from build123d import *

# Parameters (mm, degrees)
SKETCH_1_R      = 1.55
EXTRUDE_1_DEPTH = 2.1


with BuildPart() as part:
    # 草图1 → 凸台-拉伸1 (new body)
    with BuildSketch(Plane.XY):
        with BuildLine():
            Line((-13, -7.4), (13, -7.4))
            Line((13, -7.4), (13, 7.4))
            Line((13, 7.4), (7.1, 7.4))
            ThreePointArc((7.1, 7.4), (6.05, 6.35), (5, 7.4))
            Line((5, 7.4), (5, 9.5))
            Line((5, 9.5), (-5, 9.5))
            Line((-5, 9.5), (-5, 7.4))
            ThreePointArc((-5, 7.4), (-6.05, 6.35), (-7.1, 7.4))
            Line((-7.1, 7.4), (-13, 7.4))
            Line((-13, 7.4), (-13, -7.4))
        make_face()
        with BuildLine():
            ThreePointArc((-6.8, -3.05), (-7.10753788, -3.79246212), (-7.85, -4.1))
            Line((-7.85, -4.1), (-10.15, -4.1))
            ThreePointArc((-10.15, -4.1), (-11.2, -3.05), (-10.15, -2))
            Line((-10.15, -2), (-10.15, 1.8))
            ThreePointArc((-10.15, 1.8), (-11.2, 2.85), (-10.15, 3.9))
            Line((-10.15, 3.9), (-7.85, 3.9))
            ThreePointArc((-7.85, 3.9), (-7.10753788, 3.59246212), (-6.8, 2.85))
            ThreePointArc((-6.8, 2.85), (-7.10753788, 2.10753788), (-7.85, 1.8))
            Line((-7.85, 1.8), (-7.85, -2))
            ThreePointArc((-7.85, -2), (-7.10753788, -2.30753788), (-6.8, -3.05))
        make_face(mode=Mode.SUBTRACT)
        with Locations((0, 0.1)):
            Circle(SKETCH_1_R, mode=Mode.SUBTRACT)
        with BuildLine():
            ThreePointArc((7.85, 1.8), (6.8, 2.85), (7.85, 3.9))
            Line((7.85, 3.9), (10.15, 3.9))
            ThreePointArc((10.15, 3.9), (10.89246212, 3.59246212), (11.2, 2.85))
            ThreePointArc((11.2, 2.85), (10.89246212, 2.10753788), (10.15, 1.8))
            Line((10.15, 1.8), (10.15, -2))
            ThreePointArc((10.15, -2), (10.89246212, -2.30753788), (11.2, -3.05))
            ThreePointArc((11.2, -3.05), (10.89246212, -3.79246212), (10.15, -4.1))
            Line((10.15, -4.1), (7.85, -4.1))
            ThreePointArc((7.85, -4.1), (6.8, -3.05), (7.85, -2))
            Line((7.85, -2), (7.85, 1.8))
        make_face(mode=Mode.SUBTRACT)
    extrude(amount=EXTRUDE_1_DEPTH)


solid = part.part
Here's how the part is built. I have some questions about the finished solid (model axes, mm). A direction names the side the tool comes from. Coordinates: 2 decimals unless noted, no trailing zeros. Loops run counter-clockwise (first coordinate to the right, second up) from the corner with the lowest first, then second, coordinate; pieces in that order, holes last.
1. For P1, Ø0.6, axis at x = 9, z = 1, coming from the +Y side; P2, Ø0.6, axis at y = 8.5, z = 1, coming from the -X side, each with a flat end and sliding along its axis, tell me the tip position at first contact or that it passes through.
2. Imagine slicing it at A-A, the plane x = 0. Please give me the cut outline in (y, z), and give its area (3 significant figures).
3. Imagine slicing it at C-C, the plane y = 0.1. Please give me the cut outline in (x, z).
4. Imagine slicing it at D-D, the plane x = -6.05. Please give me the cut outline in (y, z).
5. I need wall thicknesses on L1, parallel to Y at x = -9.5, z = 1; L2, parallel to X at y = 1, z = 0.6; L3, parallel to Y at x = 0, z = 0.5. Which ranges of each line are inside material? Lowest first, please.
6. If we mould it in two halves opening along Y, with no side actions, what happens to faces 4 (the cylindrical face through (-0.336, -1.413, 1.035)), 5 (the flat face through (0, 3, 2.1)), 6 (the flat face through (0, -7.4, 1))? For each: pulls with the +Y half, pulls with the -Y half, needs draft (parallel to the pull), parting line crosses it, or undercut.
7. Imagine slicing it at B-B, the plane z = 1.85. Please give me the cut outline in (x, y), and give its area (3 significant figures).
8. For faces 1 (the flat face through (10.15, 0, 1)), 2 (the flat face through (13, 0, 1)), 3 (the flat face through (-5, 8, 1)), which set-ups out of +Z, -Z, +X, -X, +Y, -Y let a thin tool reach every point of the face, with its end or its side?
Taken from the geometry:
1. P1: stops at y = 7.4
1. P2: stops at x = -5
2. outline: (-7.4, 0) - (-1.45, 0) - (-1.45, 2.1) - (-7.4, 2.1) - close; (1.65, 0) - (9.5, 0) - (9.5, 2.1) - (1.65, 2.1) - close
2. area: 29.0 mm2
3. outline: (-13, 0) - (-10.15, 0) - (-10.15, 2.1) - (-13, 2.1) - close; (-7.85, 0) - (-1.55, 0) - (-1.55, 2.1) - (-7.85, 2.1) - close; (1.55, 0) - (7.85, 0) - (7.85, 2.1) - (1.55, 2.1) - close; (10.15, 0) - (13, 0) - (13, 2.1) - (10.15, 2.1) - close
4. outline: (-7.4, 0) - (6.35, 0) - (6.35, 2.1) - (-7.4, 2.1) - close
5. L1: y = -7.4 to -4.1, 3.9 to 7.4
5. L2: x = -13 to -10.15, -7.85 to -1.26, 1.26 to 7.85, 10.15 to 13
5. L3: y = -7.4 to -1.45, 1.65 to 9.5
6. face 4: undercut
6. face 5: needs draft
6. face 6: pulls with the -Y half
7. outline: (-13, -7.4) - (13, -7.4) - (13, 7.4) - (7.1, 7.4) arc R1.05 cw to (5, 7.4) - (5, 9.5) - (-5, 9.5) - (-5, 7.4) arc R1.05 cw to (-7.1, 7.4) - (-13, 7.4) - close; hole (-10.15, -4.1) - (-7.85, -4.1) arc R1.05 ccw to (-7.85, -2) - (-7.85, 1.8) arc R1.05 ccw to (-7.85, 3.9) - (-10.15, 3.9) arc R1.05 ccw to (-10.15, 1.8) - (-10.15, -2) arc R1.05 ccw to start; hole circle Ø3.1 at (0, 0.1); hole (7.85, -4.1) - (10.15, -4.1) arc R1.05 ccw to (10.15, -2) - (10.15, 1.8) arc R1.05 ccw to (10.15, 3.9) - (7.85, 3.9) arc R1.05 ccw to (7.85, 1.8) - (7.85, -2) arc R1.05 ccw to start
7. area: 344 mm2
8. face 1: +Z, -Z
8. face 2: +Z, -Z, +X, +Y, -Y
8. face 3: +Z, -Z, -X, +Y
